For this review, take the finished solid that the model builds, in its own axes (mm). A direction names the side the tool comes from. Round coordinates to 2 decimals unless told otherwise and drop trailing zeros. Order: outer loops, then holes, each group sorted by start corner. A loop starts at its lowest first (then second) coordinate and runs counter-clockwise, first axis right, second up. Notation, with made-up numbers: (82, 30) - (134, 30) arc R28 cw to (134, 52) - close; hole circle Ø3 at (2.5, 68.25). An arc over 180 degrees is marked (long way). One line per item, written item: value.
```python
from build123d import *

# Parameters (mm, degrees)
F0_W     = 60
F0_H     = 60
F1_DEPTH = 5
F2_W     = 55
F2_H     = 5
F3_DEPTH = 55
F4_R     = 25
F5_R     = 2


with BuildPart() as f1:
    # F0 (on Top) → F1 (new body)
    with BuildSketch(Plane.XY):
        Rectangle(F0_W, F0_H)
    extrude(amount=F1_DEPTH)

    # F2 (on face) → F3 (join)
    with BuildSketch(Plane.XY.offset(5)):
        Polygon((-25, 30), (-30, 30), (-30, -30), (-25, -30), (-25, 25), align=None)
        with Locations((2.5, 27.5)):
            Rectangle(F2_W, F2_H)
    extrude(amount=F3_DEPTH)

    # F4
    f4_edges = [f1.edges().sort_by_distance(p)[0] for p in [
        (30, 27.5, 60),
        (-27.5, -30, 60),
        (30, -30, 2.5),
    ]]
    fillet(f4_edges, radius=F4_R)

    # F5
    f5_edges = [f1.edges().sort_by_distance(p)[0] for p in [
        (-12.5, -30, 0),
        (22.67767, -22.67767, 0),
        (-30, 0, 0),
        (30, 12.5, 0),
        (0, 30, 0),
        (-30, 12.5, 60),
        (-30, -22.67767, 52.67767),
        (-30, 30, 30),
        (-30, -30, 17.5),
        (30, 30, 17.5),
        (22.67767, 30, 52.67767),
        (-12.5, 30, 60),
    ]]
    fillet(f5_edges, radius=F5_R)


solid = f1.part
```
Item 1: For P1, Ø8, axis at y = 16, z = 40, coming from the +X side; P2, Ø16.5, axis at x = -5, z = 38.5, coming from the -Y side; P3, Ø1.5, axis at x = 15.5, y = -17.5, coming from the +Z side, all flat-tipped, find the tip position at first contact; note any pin that passes through.
Returned:
P1: x = -25
P2: y = 25
P3: z = 5
Item 2: Take a section at A-A (z = 23). Write out the cut boundary in (x, y).
Returned:
outline: (-30, -28) arc R2 ccw to (-28, -30) - (-25, -30) - (-25, 25) - (30, 25) - (30, 28) arc R2 ccw to (28, 30) - (-28, 30) arc R2 ccw to (-30, 28) - close
Item 3: Wall thickness on line 1 (Z direction, x = -19.5, y = 19); line 2 (Y direction, x = 8, z = 44.5); line 3 (X direction, y = -24, z = 40.5): over which ranges is each line inside the solid? List them lowest first.
Returned:
line 1: 0 to 5
line 2: 25 to 30
line 3: -30 to -25
Item 4: Take a section at B-B (x = -2.5). Write out the cut boundary in (y, z), plus the area to 3 significant figures.
Returned:
outline: (-30, 2) arc R2 ccw to (-28, 0) - (28, 0) arc R2 ccw to (30, 2) - (30, 58) arc R2 ccw to (28, 60) - (25, 60) - (25, 5) - (-30, 5) - close
area: 572 mm^2
Item 5: Machinability: for faces 1 (the flat face through (2, -2, 5)), 2 (the flat face through (-30, 0, 30)), which of the approach directions +Z, -Z, +X, -X, +Y, -Y give a long, thin tool a straight path to every point of the face, cutting with its end or side? Answer none if there is none.
Returned:
face 1: +Z, +X, -Y
face 2: +Z, -Z, -X, +Y, -Y
